Can you work these out from the model? Positions are in its coordinate system, mm. Face numbers are marked on the shaded views. Give positions to 0.01 mm unless a question says otherwise; leave off trailing zeros. Loops run counter-clockwise (first coordinate to the right, second up) from the corner with the lowest first, then second, coordinate; pieces in that order, holes last. Notation, with made-up numbers: (9.25, 41) - (50.25, 41) arc R13 ccw to (50.25, 60) - close; hole circle Ø3 at (19, 14). An arc over 180 degrees is marked (long way). Write item = value, one per line.
from build123d import *

# Parameters (mm, degrees)
BOSS_EXTRUDE1_DEPTH = 0.2
FILLET1_R           = 0.3
FILLET2_R           = 0.03


with BuildPart() as part:
    # Sketch1 → Boss-Extrude1 (new body)
    with BuildSketch(Plane(origin=(0, 0, 0), x_dir=(1, 0, 0), z_dir=(0, 1, 0))):
        Polygon((0, 0), (0, 1.5), (0.65, 1.5), (0.65, 2), (2.75, 12), (2.75, 12.5), (3.25, 12.5), (3.25, 12.1), (4.05, 12.1), (4.05, 12.5), (4.55, 12.5), (4.55, 12), (6.65, 2), (6.65, 1.5), (7.3, 1.5), (7.3, 0), (6.8, 0), (6.8, 1), (6.65, 1), (6.65, 0), (0.65, 0), (0.65, 1), (0.5, 1), (0.5, 0), align=None)
    extrude(amount=BOSS_EXTRUDE1_DEPTH)

    # Fillet1
    fillet1_edges = [part.edges().sort_by_distance(p)[0] for p in [
        (0.65, 0.1, -1.5),
        (6.65, 0.1, -1.5),
    ]]
    fillet(fillet1_edges, radius=FILLET1_R)

    # Fillet2
    fillet2_edges = [part.edges().sort_by_distance(p)[0] for p in [
        (0, 0.1, 0),
        (0, 0.1, -1.5),
        (0.65, 0.1, -2),
        (2.75, 0.1, -12),
        (2.75, 0.1, -12.5),
        (3.25, 0.1, -12.5),
        (3.25, 0.1, -12.1),
        (4.05, 0.1, -12.1),
        (4.05, 0.1, -12.5),
        (4.55, 0.1, -12.5),
        (4.55, 0.1, -12),
        (6.65, 0.1, -2),
        (7.3, 0.1, -1.5),
        (7.3, 0.1, 0),
        (6.8, 0.1, 0),
        (6.8, 0.1, -1),
        (6.65, 0.1, -1),
        (6.65, 0.1, 0),
        (0.65, 0.1, 0),
        (0.65, 0.1, -1),
        (0.5, 0.1, -1),
        (0.5, 0.1, 0),
    ]]
    fillet(fillet2_edges, radius=FILLET2_R)


solid = part.part
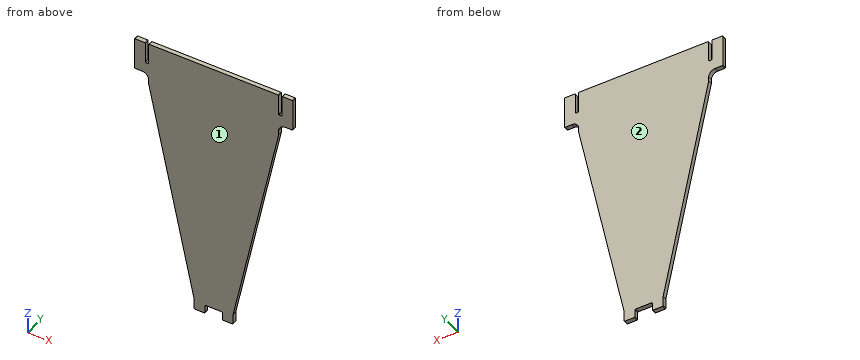
Q1. Imagine slicing it at B-B, the plane x = 5.25. Write out the boundary of the cut face in (y, z).
Output:
outline = (0, -8.67) - (0.2, -8.67) - (0.2, 0) - (0, 0) - close
Q2. We'd pull the mould along Y, two halves only. Please class the marked faces 1 and 2: released by +Y, released by -Y, zero draft, split by the parting line, or undercut.
Output:
face_1 = released by -Y
face_2 = released by +Y
Q3. I need wall thicknesses on L1, parallel to X at y = 0.1, z = -2.5 (3 decimals); L2, parallel to Z at x = 7.25, y = 0.15; L3, parallel to X at y = 0.05, z = -9.75. Which ranges of each line are inside material? Lowest first, please.
Output:
L1 = 0.755 to 6.545
L2 = -1.5 to 0
L3 = 2.28 to 5.02
Q4. Imagine slicing it at A-A, the plane z = -2.25. Write out the boundary of the cut face in (x, y).
Output:
outline = (0.7, 0) - (6.6, 0) - (6.6, 0.2) - (0.7, 0.2) - close
